Source: CAD feature listing. Evaluate the final solid. Frame: model axes, mm. A direction names the side the tool comes from. Give positions to 0.01 mm unless a question says otherwise; leave off trailing zeros. Order: outer loops, then holes, each group sorted by start corner. A loop starts at its lowest first (then second) coordinate and runs counter-clockwise, first axis right, second up.
from build123d import *

# Parameters (mm, degrees)
EXTRUDE_1_DEPTH      = 275
EXTRUDE_1_DEPTH_BACK = 270
SKETCH_1_R           = 5
SKETCH_2_R           = 3
EXTRUDE_2_DEPTH      = 15
EXTRUDE_START        = 15
SKETCH_7_R           = 3
EXTRUDE_3_DEPTH      = 15


with BuildPart() as part:
    # Эскиз1 → Бобышка-Вытянуть1 (new, two sides: drawn at the far end of the back side and taken through both)
    with BuildSketch(Plane(origin=(0, 0, 0), x_dir=(0, 0, -1), z_dir=(1, 0, 0)).offset(-EXTRUDE_1_DEPTH_BACK)):
        Circle(SKETCH_1_R)
    extrude(amount=EXTRUDE_1_DEPTH + EXTRUDE_1_DEPTH_BACK)

    # Эскиз2 → Бобышка-Вытянуть2 (add)
    with BuildSketch(Plane.ZY.offset(270)):
        Circle(SKETCH_2_R)
    extrude(amount=EXTRUDE_2_DEPTH)

    # Эскиз7 → Бобышка-Вытянуть3 (add)
    with BuildSketch(Plane(origin=(275, 0, 0), x_dir=(0, 0, -1), z_dir=(1, 0, 0)).offset(EXTRUDE_START)):
        with Locations(Location((0, 0, 0), (0, 0, 180))):
            Circle(SKETCH_7_R)
    extrude(amount=-EXTRUDE_3_DEPTH)


solid = part.part
1) First-contact query: pin 1 Ø1 at (x, y) = (79, -2) entering from +Z; pin 2 Ø1 at (x, z) = (-87, -2) entering from +Y. Flat tips, straight axial feed; report the tip coordinate or a pass-through.
Checks:
pin 1: stops at z = 4.77
pin 2: stops at y = 4.77
2) Reachability of faces 1 (the face through (275, -3.3, 0.1)), 2 (the face through (-1.31, -4.88, 1.08)), 3 (the face through (-270, -3.3, 0.1)) from +Z, -Z, +X, -X, +Y, -Y: full face, straight path, thin tool, end or side. Return the list, or none.
Checks:
face 1: +X
face 2: +X, -X
face 3: -X
3) Section query C-C on x = 253. Output: boundary loops of the cut face in (y, z).
Checks:
outline: circle Ø10 at (0, 0)
4) Section query A-A on y = 0. Output: boundary loops of the cut face in (x, z), and give its area (3 significant figures).
Checks:
outline: (-285, -3) - (-270, -3) - (-270, -5) - (275, -5) - (275, -3) - (290, -3) - (290, 3) - (275, 3) - (275, 5) - (-270, 5) - (-270, 3) - (-285, 3) - close
area: 5,630 mm2
5) Ray query, L1, parallel to X at y = -4, z = -1.5; L2, parallel to Y at x = -3, z = 0.75; L3, parallel to Z at x = -156, y = 0.5. Return the intervals inside material, ascending.
Checks:
L1: x = -270 to 275
L2: y = -4.94 to 4.94
L3: z = -4.97 to 4.97
